Drawing for the job (mm, zero at the part's lowest x, y, z). A direction names the side the tool comes from. Round coordinates to 2 decimals unless told otherwise and drop trailing zeros. Order: outer loops, then holes, each group sorted by start corner. A loop starts at its lowest first (then second) coordinate and runs counter-clockwise, first axis right, second up. Notation, with made-up numbers: (39.5, -29.5) - (92.5, -29.5) arc R22 ccw to (92.5, -5.5) - close; hole circle Ø10 at (81, 5.5). An arc over 180 degrees is marked (long way). Answer as a JSON object with one key per item and string values.
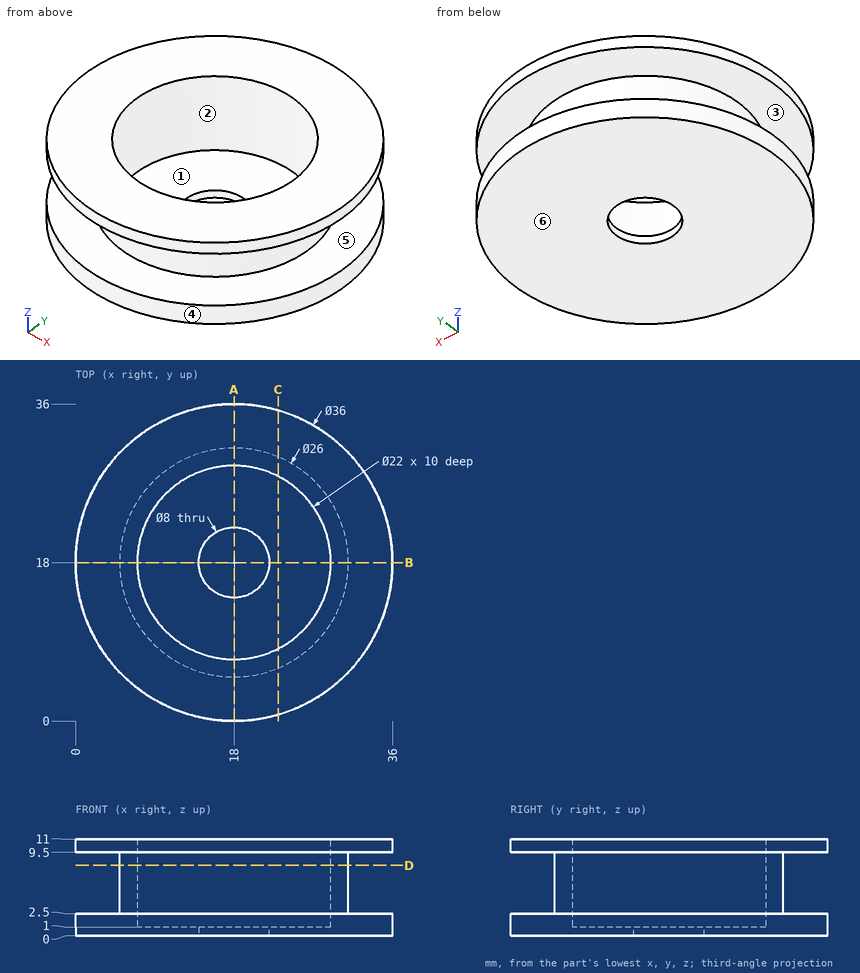
Item 1: Drop flat-ended pins along their axis: P1, Ø4, axis at y = 16, z = 9.5, coming from the -X side; P2, Ø2, axis at x = 6.5, z = 6, coming from the -Y side; P3, Ø5, axis at x = 16.5, z = 5.5, coming from the -Y side; P4, Ø1, axis at y = 9, z = 2.5, coming from the +X side. Give the stop position or say it passes through.
Taken from the geometry:
{"P1": "x = 0", "P2": "y = 10.34", "P3": "y = 5", "P4": "x = 33.87"}
Item 2: Probe L1, parallel to Z at x = 21, y = 31.5; L2, parallel to Y at x = 18, z = 4.5; L3, parallel to Y at x = 18, z = 0.3. List the from-to ranges inside material, lowest first. Write a range as from..to.
Taken from the geometry:
{"L1": "0..2.5, 9.5..11", "L2": "5..7, 29..31", "L3": "0..14, 22..36"}
Item 3: Two-plate mould, pull along Y, no slides. Class the marked faces 1, 2, 3 and 4: pulls with the +Y half, pulls with the -Y half, needs draft (parallel to the pull), parting line crosses it, or undercut.
Taken from the geometry:
{"face 1": "undercut", "face 2": "undercut", "face 3": "needs draft", "face 4": "parting line crosses it"}
Item 4: Cut at D-D (z = 8). Write the cut outline in (x, y).
Taken from the geometry:
{"outline": "circle Ø26 at (18, 18); hole circle Ø22 at (18, 18)"}
Item 5: Cut at A-A (x = 18). Write the cut outline in (y, z), plus the area to 3 significant figures.
Taken from the geometry:
{"outline": "(0, 0) - (14, 0) - (14, 1) - (7, 1) - (7, 11) - (0, 11) - (0, 9.5) - (5, 9.5) - (5, 2.5) - (0, 2.5) - close; (22, 0) - (36, 0) - (36, 2.5) - (31, 2.5) - (31, 9.5) - (36, 9.5) - (36, 11) - (29, 11) - (29, 1) - (22, 1) - close", "area": "98.0 mm2"}
Item 6: Tool access for the marked faces 5 and 6: list every direction of +Z, -Z, +X, -X, +Y, -Y with a clear straight run to the whole face (end or side of a thin tool).
Taken from the geometry:
{"face 5": "none", "face 6": "-Z, +X, -X, +Y, -Y"}
Item 7: Cut at C-C (x = 23). Write the cut outline in (y, z), plus the area to 3 significant figures.
Taken from the geometry:
{"outline": "(0.71, 0) - (35.29, 0) - (35.29, 2.5) - (30, 2.5) - (30, 9.5) - (35.29, 9.5) - (35.29, 11) - (27.8, 11) - (27.8, 1) - (8.2, 1) - (8.2, 11) - (0.71, 11) - (0.71, 9.5) - (6, 9.5) - (6, 2.5) - (0.71, 2.5) - close", "area": "110 mm2"}
